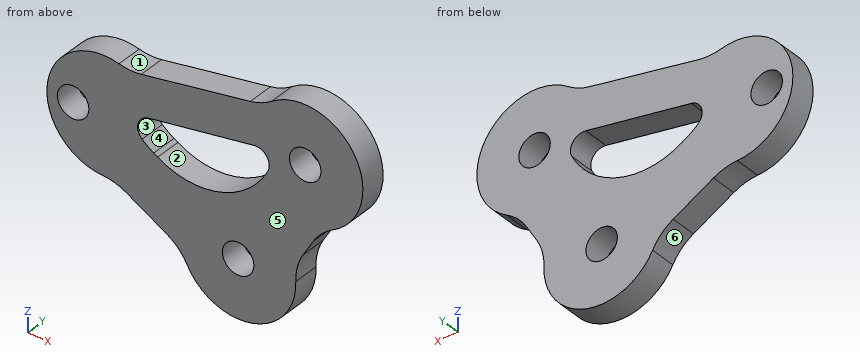
from build123d import *

# Parameters (mm, degrees)
SKETCH1_R           = 6
BOSS_EXTRUDE1_DEPTH = 10


with BuildPart() as part:
    # Sketch1 → Boss-Extrude1 (new body)
    with BuildSketch(Plane(origin=(0, 0, 0), x_dir=(1, 0, 0), z_dir=(0, 1, 0))):
        with BuildLine():
            Line((42.951232399, 3.318887452), (39.045860783, 9.872476959))
            ThreePointArc((39.045860783, 9.872476959), (36.854758208, 15.13768422), (36.238749427, 20.807240744))
            ThreePointArc((36.238749427, 20.807240744), (19.926498256, 42.82902865), (-5.191028063, 31.867342993))
            ThreePointArc((-5.191028063, 31.867342993), (-8.539203816, 27.271038576), (-13.045616394, 23.802819891))
            Line((-13.045616394, 23.802819891), (-28.400215901, 15.147576948))
            ThreePointArc((-28.400215901, 15.147576948), (-32.789279464, 13.321988508), (-37.485200727, 12.583763884))
            ThreePointArc((-37.485200727, 12.583763884), (-58.444412115, -12.582400357), (-31.160339611, -30.698794925))
            ThreePointArc((-31.160339611, -30.698794925), (-26.9348971, -30.075669304), (-22.673496589, -30.363967139))
            Line((-22.673496589, -30.363967139), (18.895945155, -37.693778855))
            ThreePointArc((18.895945155, -37.693778855), (23.162809039, -38.948266928), (27.046941071, -41.114689344))
            ThreePointArc((27.046941071, -41.114689344), (58.445846615, -34.941068913), (50.465944263, -3.951941513))
            ThreePointArc((50.465944263, -3.951941513), (46.22501506, -0.816320632), (42.951232399, 3.318887452))
        make_face()
        with Locations(Location((-48.675608258, -9.401334707, 0), (0, 0, 270))):
            Circle(SKETCH1_R, mode=Mode.SUBTRACT)
        with Locations(Location((14.252094878, 21.573414185, 0), (0, 0, 270))):
            Circle(SKETCH1_R, mode=Mode.SUBTRACT)
        with Locations(Location((39.833295256, -23.211920099, 0), (0, 0, 270))):
            Circle(SKETCH1_R, mode=Mode.SUBTRACT)
        with BuildLine():
            Line((20.312704962, -22.212607301), (-19.891412958, -15.548077687))
            ThreePointArc((-19.891412958, -15.548077687), (-23.883928025, -11.979955979), (-22.359792068, -6.846859578))
            ThreePointArc((-22.359792068, -6.846859578), (-20.208737863, -5.13808357), (-17.910389919, -3.633242594))
            Line((-17.910389919, -3.633242594), (-16.434238636, -2.760580859))
            ThreePointArc((-16.434238636, -2.760580859), (7.233462597, 0.214394926), (25.58991918, -15.018827461))
            ThreePointArc((25.58991918, -15.018827461), (25.161933747, -20.2373856), (20.312704962, -22.212607301))
        make_face(mode=Mode.SUBTRACT)
    extrude(amount=BOSS_EXTRUDE1_DEPTH)


solid = part.part
Geometry: final body of the model. Coordinates: model frame, mm. Face numbers are marked on the shaded views. A direction names the side the tool comes from. Coordinates: 2 decimals unless noted, no trailing zeros. Loops run counter-clockwise (first coordinate to the right, second up) from the corner with the lowest first, then second, coordinate; pieces in that order, holes last. Notation, with made-up numbers: (57.25, 75) - (93.25, 75) arc R22 ccw to (93.25, 91) - close; hole circle Ø6 at (-32.5, 46). An arc over 180 degrees is marked (long way). One line per question, with ' | ' between items. Start each with the question number.
(1) Cut plane A-A on x = 3. Output: boundary loops of the cut face in (y, z).
(2) Cut plane D-D on x = 17.5. Output: boundary loops of the cut face in (y, z).
(3) Cut plane C-C on y = 8.25. Output: boundary loops of the cut face in (x, z).
(4) Reachability of the marked faces 1 and 2 from +Z, -Z, +X, -X, +Y, -Y: full face, straight path, thin tool, end or side. Return the list, or none.
(5) Draft query along X for the marked faces 3, 4, 5 and 6. Return one class per face: +X half, -X half, draft (parallel to the pull), parting line (faces both ways), or undercut.
(6) First-contact query: pin 1 (11 mm diameter, centred on x = 14.25, z = -21.57, fed in from +Y); pin 2 (2 mm diameter, centred on y = 4.5, z = -5, fed in from -X); pin 3 (15.5 mm diameter, centred on x = 39.83, z = 23.21, fed in from -Y); pin 4 (4 mm diameter, centred on x = -24, y = 5.5, fed in from -Z). Flat tips, straight axial feed; report the tip coordinate or a pass-through.
(7) Cut plane B-B on z = -18. Output: boundary loops of the cut face in (x, y).
(8) Ray query, L1, parallel to X at y = 3.75, z = 7.5; L2, parallel to X at y = 8.25, z = 9.5; L3, parallel to Z at x = -3, y = 8. Return the intervals inside material, ascending. Write a range as from..to.
Here are the results:
1) outline: (0, -40.48) - (10, -40.48) - (10, -1.12) - (0, -1.12) - close; (0, 19.34) - (10, 19.34) - (10, 34.89) - (0, 34.89) - close
2) outline: (0, -43.33) - (10, -43.33) - (10, -26.62) - (0, -26.62) - close; (0, -16.53) - (10, -16.53) - (10, 5.1) - (0, 5.1) - close; (0, 21.75) - (10, 21.75) - (10, 37.45) - (0, 37.45) - close
3) outline: (-37.49, -12.58) arc R20 cw to (-28.4, -15.15) - (-13.05, -23.8) arc R20 cw to (-5.19, -31.87) arc R22 ccw to (36.24, -20.81) arc R20 cw to (39.05, -9.87) - (42.95, -3.32) arc R20 cw to (50.47, 3.95) arc R22 ccw (long way) to (27.05, 41.11) arc R20 cw to (18.9, 37.69) - (-22.67, 30.36) arc R20 cw to (-31.16, 30.7) arc R22 ccw (long way) to start; hole circle Ø12 at (-48.68, 9.4); hole (-22.36, 6.85) arc R30 ccw to (-17.91, 3.63) - (-16.43, 2.76) arc R30 ccw to (25.59, 15.02) arc R5 ccw to (20.31, 22.21) - (-19.89, 15.55) arc R5 ccw to start; hole circle Ø12 at (14.25, -21.57); hole circle Ø12 at (39.83, 23.21)
4) face 1: +Z, +Y, -Y | face 2: +Y, -Y
5) face 3: undercut | face 4: undercut | face 5: draft | face 6: -X half
6) pin 1: through | pin 2: x = -54.12 | pin 3: y = 0 | pin 4: z = -18.76
7) outline: (-23.34, 0) - (9.43, 0) - (9.43, 10) - (-23.34, 10) - close; (19.07, 0) - (36.34, 0) - (36.34, 10) - (19.07, 10) - close
8) L1: -58.59..-54.37, -42.98..-22.98, 20.17..55.23 | L2: -58.68..-54.67, -42.68..-23.95, 21.98..57.04 | L3: -35.22..-1.36, 18.35..33.83
